Can you work these out from the model? Positions are in its coordinate system, mm. Give positions to 0.01 mm unless a question says otherwise; leave off trailing zeros. Order: outer loops, then holes, each group sorted by start corner. A loop starts at its lowest first (then second) coordinate and runs counter-clockwise, first axis right, second up. Notation, with made-up numbers: (-37.75, 79.5) - (-10.75, 79.5) arc R16 ccw to (-10.75, 87.5) - close; hole circle Ø11 at (54.25, -2.75). An arc over 180 degrees is marked (long way). Answer as CSV lines item,"result".
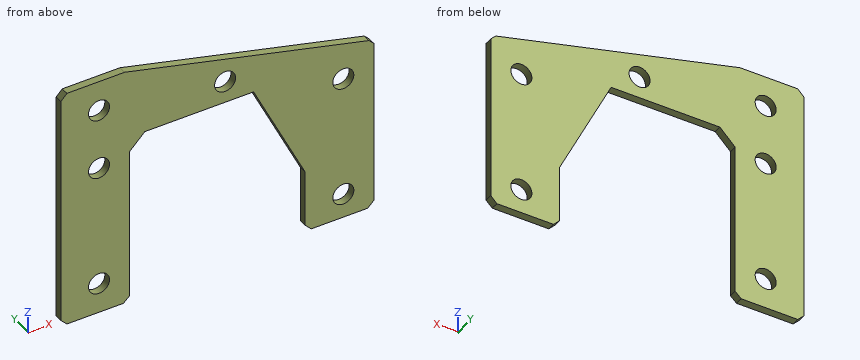
Autodesk Inventor part; units mm, degrees
ref_plane "YZ Plane" through (0, 0, 0) normal (1, 0, 0) x (0, 1, 0)
ref_plane "XZ Plane" through (0, 0, 0) normal (0, 1, 0) x (-1, 0, 0)
ref_plane "XY Plane" through (0, 0, 0) normal (0, 0, 1) x (1, 0, 0)
sketch "Sketch1" plane through (0, 0, 0) normal (0, 1, 0) x (-1, 0, 0)
  circle A0 centre (28.5676, 25.8614) radius 2.1844
  circle A1 centre (28.5676, -12.2386) radius 2.1844
  circle A2 centre (28.5676, 13.1614) radius 2.1844
  circle A3 centre (-22.2324, -12.2386) radius 2.1844
  circle A4 centre (-22.2324, 13.1614) radius 2.1844
  line L0 (23.2336, 32.2114) -> (-27.5664, 19.5114)
  line L1 (-27.5664, 19.5114) -> (-28.5824, 18.4954)
  line L2 (23.2336, 32.2114) -> (34.1239, 32.2114)
  line L3 (35.2397, -18.5886) -> (23.4876, -18.5886)
  line L4 (36.5097, 30.9154) -> (36.5097, -17.3186)
  line L5 (22.2214, 14.3333) -> (22.2214, -17.4167)
  line L6 (19.0464, 17.5083) -> (-2.1664, 17.5083)
  line L7 (-14.2949, -16.0486) -> (-15.5649, -17.3186)
  line L8 (-27.3124, -17.3186) -> (-28.5824, -16.0486)
  line L9 (22.2214, 14.3333) -> (19.0464, 17.5083)
  line L10 (36.5097, 30.9154) -> (35.24, 32.2114)
  line L11 (36.5097, -17.3186) -> (35.2397, -18.5886)
  line L12 (23.4876, -18.5886) -> (22.2214, -17.4167)
  line L13 (35.24, 32.2114) -> (34.1239, 32.2114)
  line L14 (-15.5649, -17.3186) -> (-27.3124, -17.3186)
  line L15 (-28.5824, -16.0486) -> (-28.5824, 18.4954)
  line L16 (-14.2949, -12.2386) -> (-14.2949, -16.0486)
  line L17 (-14.2949, -12.2386) -> (-14.2949, -4.3011)
  line L18 (-3.5693, 17.5083) -> (-14.2949, -4.3011)
  line L19 (-2.1664, 17.5083) -> (-3.5693, 17.5083)
  circle A5 centre (2.3498, 22.0704) radius 2.1844
  point P0 (0, 0)
  point P1 (36.5051, 32.2114)
  dimension "d0" = 31.75
  dimension "d6" = 4.3688
extrude "Extrusion1" add sketch "Sketch1" along normal blind 1.5875
properties part number "backFunnel"
1) I want a section at D-D on x = -1. Write out the boundary of the cut face in (y, z), plus the area to 3 significant figures.
Answer block:
outline,"(0, 17.51) - (1.59, 17.51) - (1.59, 20.35) - (0, 20.35) - close; (0, 23.79) - (1.59, 23.79) - (1.59, 26.65) - (0, 26.65) - close"
area,"9.06 mm2"
2) I want a section at B-B on z = 16.5. Write out the boundary of the cut face in (x, y), plus the area to 3 significant figures.
Answer block:
outline,"(-36.51, 0) - (-20.05, 0) - (-20.05, 1.59) - (-36.51, 1.59) - close; (4.07, 0) - (28.58, 0) - (28.58, 1.59) - (4.07, 1.59) - close"
area,"65.0 mm2"
3) I want a section at C-C on y = 0.7. Write out the boundary of the cut face in (x, z).
Answer block:
outline,"(-36.51, -17.32) - (-35.24, -18.59) - (-23.49, -18.59) - (-22.22, -17.42) - (-22.22, 14.33) - (-19.05, 17.51) - (3.57, 17.51) - (14.29, -4.3) - (14.29, -16.05) - (15.56, -17.32) - (27.31, -17.32) - (28.58, -16.05) - (28.58, 18.5) - (27.57, 19.51) - (-23.23, 32.21) - (-35.24, 32.21) - (-36.51, 30.92) - close; hole circle Ø4.37 at (-28.57, -12.24); hole circle Ø4.37 at (-28.57, 13.16); hole circle Ø4.37 at (-28.57, 25.86); hole circle Ø4.37 at (-2.35, 22.07); hole circle Ø4.37 at (22.23, -12.24); hole circle Ø4.37 at (22.23, 13.16)"
4) I want a section at A-A on x = 22.5. Write out the boundary of the cut face in (y, z), plus the area to 3 significant figures.
Answer block:
outline,"(0, -17.32) - (1.59, -17.32) - (1.59, -14.41) - (0, -14.41) - close; (0, -10.07) - (1.59, -10.07) - (1.59, 10.99) - (0, 10.99) - close; (0, 15.33) - (1.59, 15.33) - (1.59, 20.78) - (0, 20.78) - close"
area,"46.7 mm2"
5) I need wall thicknesses on line 1 along X through (y, z) = (1.25, -7); line 2 along X through (y, z) = (0.55, -11); line 3 along X through (y, z) = (0.2, 12.5). Which ranges of each line are inside material? Lowest first, please. Write a range as [from, to].
Answer block:
line 1,"[-36.51, -22.22], [14.29, 28.58]"
line 2,"[-36.51, -30.37], [-26.77, -22.22], [14.29, 20.43], [24.03, 28.58]"
line 3,"[-36.51, -30.65], [-26.49, -22.22], [6.03, 20.15], [24.31, 28.58]"
